```python
from build123d import *

# Parameters (mm, degrees)
F0_R     = 11.25
F0_R_2   = 6.25
F0_R_3   = 15
F1_DEPTH = 5
F2_DEPTH = 1.5
F3_DEPTH = 2


with BuildPart() as f1:
    # F0 (on Top) → F1 (new body)
    with BuildSketch(Plane.XY):
        with BuildLine():
            ThreePointArc((3.34966, 55.296498), (0.858471, 50.413827), (0, 45))
            Line((0, 45), (0, 17.5))
            ThreePointArc((0, 17.5), (5.125631, 5.125631), (17.5, 0))
            Line((17.5, 0), (127.5, 0))
            ThreePointArc((127.5, 0), (139.874369, 5.125631), (145, 17.5))
            Line((145, 17.5), (145, 45))
            ThreePointArc((145, 45), (143.800402, 50.302852), (141.65034, 55.296498))
            Line((141.65034, 55.296498), (133.144315, 66.986215))
            ThreePointArc((133.144315, 66.986215), (106.525074, 89.696187), (72.5, 97.858366))
            ThreePointArc((72.5, 97.858366), (38.474926, 89.696187), (11.855685, 66.986215))
            Line((11.855685, 66.986215), (3.34966, 55.296498))
        make_face()
        with Locations((17.5, 17.5)):
            Circle(F0_R, mode=Mode.SUBTRACT)
        with Locations((45, 17.5)):
            Circle(F0_R, mode=Mode.SUBTRACT)
        with Locations((17.5, 45)):
            Circle(F0_R, mode=Mode.SUBTRACT)
        with Locations((45, 45)):
            Circle(F0_R, mode=Mode.SUBTRACT)
        with Locations((72.5, 17.5)):
            Circle(F0_R, mode=Mode.SUBTRACT)
        with Locations((100, 17.5)):
            Circle(F0_R, mode=Mode.SUBTRACT)
        with Locations((127.5, 17.5)):
            Circle(F0_R, mode=Mode.SUBTRACT)
        with Locations((72.5, 45)):
            Circle(F0_R, mode=Mode.SUBTRACT)
        with Locations((100, 45)):
            Circle(F0_R, mode=Mode.SUBTRACT)
        with Locations((127.5, 45)):
            Circle(F0_R, mode=Mode.SUBTRACT)
        with Locations((27.093764, 68.08592)):
            Circle(F0_R_2, mode=Mode.SUBTRACT)
        with Locations((55, 75)):
            Circle(F0_R_3, mode=Mode.SUBTRACT)
        with Locations((117.906236, 68.08592)):
            Circle(F0_R_2, mode=Mode.SUBTRACT)
        with Locations((90, 75)):
            Circle(F0_R_3, mode=Mode.SUBTRACT)
    extrude(amount=F1_DEPTH)

    # F0 (on Top) → F2 (join)
    with BuildSketch(Plane.XY):
        with Locations((55, 75)):
            Circle(F0_R_3)
        with Locations((90, 75)):
            Circle(F0_R_3)
    extrude(amount=F2_DEPTH)

    # F0 (on Top) → F3 (join)
    with BuildSketch(Plane.XY):
        with Locations((17.5, 45)):
            Circle(F0_R)
        with Locations((17.5, 17.5)):
            Circle(F0_R)
        with Locations((45, 45)):
            Circle(F0_R)
        with Locations((45, 17.5)):
            Circle(F0_R)
        with Locations((72.5, 45)):
            Circle(F0_R)
        with Locations((72.5, 17.5)):
            Circle(F0_R)
        with Locations((100, 45)):
            Circle(F0_R)
        with Locations((100, 17.5)):
            Circle(F0_R)
        with Locations((127.5, 45)):
            Circle(F0_R)
        with Locations((127.5, 17.5)):
            Circle(F0_R)
    extrude(amount=F3_DEPTH)


solid = f1.part
```
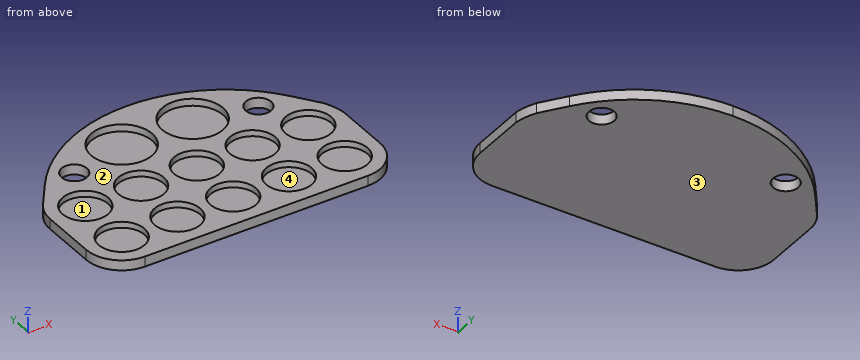
Part model, mm, in its own coordinate system. Face numbers are marked on the shaded views. A direction names the side the tool comes from. Coordinates: 2 decimals unless noted, no trailing zeros. Order: outer loops, then holes, each group sorted by start corner. A loop starts at its lowest first (then second) coordinate and runs counter-clockwise, first axis right, second up. Notation, with made-up numbers: (-27.5, 64.25) - (18.5, 64.25) arc R25 ccw to (18.5, 103.25) - close; hole circle Ø4 at (45, 76). An arc over 180 degrees is marked (long way). Return JSON: item names as keys, results as strings. Group by question number.
Item 1: Which spindle directions (+Z, -Z, +X, -X, +Y, -Y) get a long thin tool onto all of the face, cutting with end or side? Do the marked faces 3 and 4. Say none if no direction does.
Item 2: Cut at B-B (x = 93.5). List the corners of the cut face in (y, z).
Item 3: Pull direction X, two halves, no side cores. Call the marked faces 1 and 2: pulls with the +X half, pulls with the -X half, needs draft (parallel to the pull), parting line crosses it, or undercut.
Item 4: Cut at A-A (y = 70). List the corners of the cut face in (x, z).
Item 5: Pin check, flat tips, straight feed: pin 1 (11 mm diameter, centred on x = 101, y = 14.5, fed in from +Z); pin 2 (3 mm diameter, centred on y = 74.5, z = 4.5, fed in from +X); pin 3 (1 mm diameter, centred on x = 100, y = 73, fed in from +Z). Stop position of each tip, or through.
Item 6: Cut at C-C (y = 43). List the corners of the cut face in (x, z).
Item 7: Cut at D-D (x = 45). List the corners of the cut face in (y, z).
Item 8: Drill centre lines: probe 1 along Y at (x, z) = (45.5, 2.95); probe 2 along Y at (x, z) = (136.5, 3.3); probe 3 along Y at (x, z) = (123.5, 3.35). Where is each one in solid material? Low to high. Write a range as from..to.
Check values:
{
 "1": {"face 3": "-Z, +X, -X, +Y, -Y", "face 4": "+Z"},
 "2": {"outline": "(0, 0) - (94.86, 0) - (94.86, 5) - (89.59, 5) - (89.59, 1.5) - (60.41, 1.5) - (60.41, 5) - (54.18, 5) - (54.18, 2) - (35.82, 2) - (35.82, 5) - (26.68, 5) - (26.68, 2) - (8.32, 2) - (8.32, 5) - (0, 5) - close"},
 "3": {"face 1": "undercut", "face 2": "needs draft"},
 "4": {"outline": "(14.17, 0) - (21.14, 0) - (21.14, 5) - (14.17, 5) - close; (33.04, 0) - (111.96, 0) - (111.96, 5) - (104.14, 5) - (104.14, 1.5) - (75.86, 1.5) - (75.86, 5) - (69.14, 5) - (69.14, 1.5) - (40.86, 1.5) - (40.86, 5) - (33.04, 5) - close; (123.86, 0) - (130.83, 0) - (130.83, 5) - (123.86, 5) - close"},
 "5": {"pin 1": "stops at z = 2", "pin 2": "stops at x = 128.27", "pin 3": "stops at z = 1.5"},
 "6": {"outline": "(0, 0) - (145, 0) - (145, 5) - (138.57, 5) - (138.57, 2) - (116.43, 2) - (116.43, 5) - (111.07, 5) - (111.07, 2) - (88.93, 2) - (88.93, 5) - (83.57, 5) - (83.57, 2) - (61.43, 2) - (61.43, 5) - (56.07, 5) - (56.07, 2) - (33.93, 2) - (33.93, 5) - (28.57, 5) - (28.57, 2) - (6.43, 2) - (6.43, 5) - (0, 5) - close"},
 "7": {"outline": "(0, 0) - (92.63, 0) - (92.63, 5) - (86.18, 5) - (86.18, 1.5) - (63.82, 1.5) - (63.82, 5) - (56.25, 5) - (56.25, 2) - (33.75, 2) - (33.75, 5) - (28.75, 5) - (28.75, 2) - (6.25, 2) - (6.25, 5) - (0, 5) - close"},
 "8": {"probe 1": "y = 0..6.26, 28.74..33.76, 56.24..63.39, 86.61..92.83", "probe 2": "y = 2.49..10.75, 24.25..38.25, 51.75..62.37", "probe 3": "y = 0..6.99, 28.01..34.49, 55.51..65.3, 70.87..77.85"}
}
